Autodesk Inventor part; units mm, degrees
ref_plane "YZ Plane" through (0, 0, 0) normal (1, 0, 0) x (0, 1, 0)
ref_plane "XZ Plane" through (0, 0, 0) normal (0, 1, 0) x (-1, 0, 0)
ref_plane "XY Plane" through (0, 0, 0) normal (0, 0, 1) x (1, 0, 0)
sketch "Sketch1" plane through (0, 0, 0) normal (1, 0, 0) x (0, 1, 0)
  line L0 (0, 0) -> (158.3288, -141.2692)
  line L1 (155, -150) -> (0, -150)
  line L2 (0, -150) -> (0, 0)
  arc A0 (155, -150) -> (158.3288, -141.2692) centre (155, -145) ccw
  point P0 (168.114, -150)
  dimension "d1" = 150
  dimension "d2" = 5
  dimension "d3" = 155
extrude "Extrusion1" add sketch "Sketch1" along normal mid plane 15
fillet "Fillet1" radius 5 6 edges at (7.5, 159.6719, -146.7813) (7.5, 77.5, -150) (7.5, 79.1644, -70.6346) (-7.5, 159.6719, -146.7813) (-7.5, 77.5, -150) (-7.5, 79.1644, -70.6346)
properties part number "Wing_vertical"
The model under review builds one solid part; all positions refer to its coordinate system, in mm. Round coordinates to 2 decimals unless told otherwise and drop trailing zeros. Order: outer loops, then holes, each group sorted by start corner. A loop starts at its lowest first (then second) coordinate and runs counter-clockwise, first axis right, second up. Notation, with made-up numbers: (13.25, 6) - (56.25, 6) arc R28 cw to (56.25, 33) - close; hole circle Ø7 at (85, 63.25). An arc over 180 degrees is marked (long way). Use one line per item in the form item = value.
Q1. Add section A-A on x = -0.5. Give the boundary of the cut face in (y, z), then the cut area to 3 significant figures.
Response values:
outline = (0, -150) - (155, -150) arc R5 ccw to (158.33, -141.27) - (0, 0) - close
area = 12,600 mm^2
Q2. Clearance check with flat-ended pins moving along their axes: P1, Ø1.5, axis at x = 3.5, y = 54.5, coming from the -Z side; P2, Ø3, axis at y = 114.5, z = -106.5, coming from the +X side; P3, Ø1, axis at x = 5.5, y = 77, coming from the -Z side. State where each tip first meets the part, or that it passes through.
Response values:
P1 = -149.99
P2 = 7.49
P3 = -149.33
Q3. To check wall thickness, follow line 1 (Z direction, x = -4.75, y = 93.5); line 2 (Z direction, x = -6.25, y = 127.5); line 3 (Y direction, x = 0.75, z = -86.5). State the ranges of each line that lie inside material, in increasing order.
Response values:
line_1 = -149.47 to -84.14
line_2 = -148.31 to -116.03
line_3 = 0 to 96.95
Q4. Mouldability with a two-part tool opening along X and no side actions: class faces 1 (the flat face through (7.5, 59, -90)), 2 (the flat face through (0, 79, -150)), 3 (the cylindrical face through (-5.996, 77.107, -70.71)) as pulls with the +X half, pulls with the -X half, needs draft (parallel to the pull), parting line crosses it, or undercut.
Response values:
face_1 = pulls with the +X half
face_2 = needs draft
face_3 = pulls with the -X half
